The listing builds one solid part. Answer for the finished solid, in the listing's coordinates (mm). A direction names the side the tool comes from. Coordinates: 2 decimals unless noted, no trailing zeros. Order: outer loops, then holes, each group sorted by start corner. A loop starts at its lowest first (then second) coordinate and runs counter-clockwise, first axis right, second up. Notation, with made-up numbers: (81.5, 80) - (115.5, 80) arc R27 cw to (115.5, 106) - close; hole circle Ø8 at (67, 86.5). An arc over 180 degrees is marked (long way). Use one line per item in the form item = value. Start each with the question number.
Item 1: Each of these flat-tipped pins is pushed along its axis until it touches: pin 1 Ø4 at (x, z) = (-3, 39) entering from +Y; pin 2 Ø1 at (y, z) = (-4, 14) entering from -X; pin 3 Ø1.4 at (x, y) = (-5, -1) entering from -Z; pin 4 Ø1.5 at (y, z) = (-3.5, 42.5) entering from -X. Where does it stop, or does it pass through?
Item 2: Section B-B, the plane x = 7.25 is taken. Write down the section's boundary in (y, z).
Item 3: Section C-C, the plane y = -4.5 is taken. Write down the section's boundary in (x, z), and give its area (3 significant figures).
Item 4: A tool of negligible diameter and unlimited length cuts with its end or side. For faces 1 (the flat face through (5, 2.54, 7)), 2 (the flat face through (-4, 2.54, 6)), 3 (the flat face through (-4, -2.54, 6)), 4 (the cylindrical face through (-1.106, -5.814, 19.709)), 5 (the flat face through (3, 2, 38.1)), from which of +Z, -Z, +X, -X, +Y, -Y can it reach the whole face along a straight path? Write none if from no direction.
Item 5: Consider line 1 along Z through (x, y) = (3, 2); line 2 along Y through (x, z) = (3.75, 10); line 3 along X through (y, z) = (-3.5, 28). Determine where each line is inside the solid, lowest interval first. Write a range as [from, to].
Item 6: Section A-A, the plane z = 35.5 is taken. Write down the section's boundary in (x, y).
from build123d import *

# Parameters (mm, degrees)
F0_R     = 4
F1_DEPTH = 38.1
F5_DEPTH = 2.54
F7_R     = 1.5
F8_DEPTH = 4.064


with BuildPart() as f1:
    # F0 (on Top) → F1 (new body)
    with BuildSketch(Plane.XY):
        Circle(F0_R)
    extrude(amount=F1_DEPTH)

    # F2 (on Right) → F3 (revolve)
    with BuildSketch(Plane.YZ):
        Polygon((0, 50.466843), (0, 36.88176), (3.484131, 38.298216), align=None)
    revolve(axis=Axis((0, 0, 43.674301), (0, 0, 1)))

    # F4 (on Front) → F5 (join, symmetric)
    with BuildSketch(Plane.XZ):
        Polygon((-7.716181, 2.000377), (-2.643188, 2.000377), (-3.163495, 15.008056), align=None)
        Polygon((7.716181, 2.000377), (3.163495, 15.008056), (2.643188, 2.000377), align=None)
    extrude(amount=F5_DEPTH, both=True)

    # F7 (on offset) → F8 (join)
    with BuildSketch(Plane.XZ.offset(3.81)):
        with Locations((0, 18.695335)):
            Circle(F7_R)
    extrude(amount=F8_DEPTH)


solid = f1.part
Response:
q1.pin_1 = 3.81
q1.pin_2 = -1.94
q1.pin_3 = 2
q1.pin_4 = through
q2.outline = (-2.54, 2) - (2.54, 2) - (2.54, 3.33) - (-2.54, 3.33) - close
q3.outline = circle Ø3 at (0, 18.7)
q3.area = 7.07 mm2
q4.face_1 = +Z, -Z, +X, +Y
q4.face_2 = +Z, -Z, -X, +Y
q4.face_3 = +Z, -Z, -X, -Y
q4.face_4 = -Y
q4.face_5 = none
q5.line_1 = [0, 38.1]
q5.line_2 = [-2.54, 2.54]
q5.line_3 = [-1.94, 1.94]
q6.outline = circle Ø8 at (0, 0)
